For this review, take the finished solid that the model builds, in its own axes (mm). Face numbers are marked on the shaded views. A direction names the side the tool comes from. Coordinates: 2 decimals unless noted, no trailing zeros. Write each loop counter-clockwise with the first axis right and the second up, starting at its lowest first coordinate (ties: lowest second). Pieces come first, ordered by that corner, then holes.
1) Mouldability with a two-part tool opening along Z and no side actions: class the marked faces 5, 6 and 7 as pulls with the +Z half, pulls with the -Z half, needs draft (parallel to the pull), parting line crosses it, or undercut.
2) Insertion check: P1, Ø3, axis at y = 15, z = 25, coming from the -X side (3 decimals); P2, Ø3, axis at x = 24.5, z = 20.5, coming from the -Y side; P3, Ø12, axis at x = 38.5, z = 27, coming from the +Y side; P4, Ø8, axis at y = 41.5, z = 32.5, coming from the -X side. Each pin has a flat end and moves straight along its axis. Give the tip position at first contact, or say it passes through.
3) We need section C-C on y = 21.5. Write out the cut boundary in (x, z) (3 decimals), then the cut area to 3 significant figures.
4) We need section D-D on x = 102.5. Write out the cut boundary in (y, z) (3 decimals).
5) For the marked faces 1, 2, 3 and 4, list the 3-axis set-ups (+Z, -Z, +X, -X, +Y, -Y) from which the entire face can be reached by the end or side of a thin tool; tool diameter is ignored.
6) We need section B-B on x = 43. Write out the cut boundary in (y, z) (3 decimals).
7) To check wall thickness, follow line 1 along Z through (x, y) = (6, 47) (3 decimals); line 2 along X through (y, z) = (-34, 3.5) (3 decimals); line 3 along Y through (x, z) = (11.5, 22). State the ranges of each line that lie inside material, in increasing order.
8) We need section A-A on y = -47.5. Write out the cut boundary in (x, z) (3 decimals).
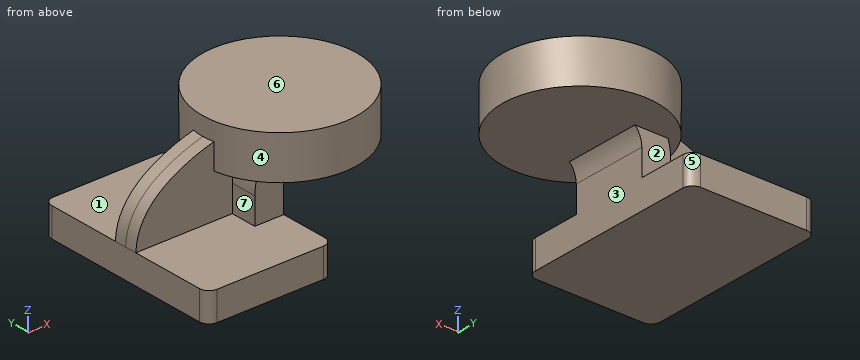
from build123d import *

# Parameters (mm, degrees)
F1_DEPTH = 63.5
F2_DEPTH = 25.4
F3_DEPTH = 7.9375
F5_R     = 6.35


with BuildPart() as f1:
    # F0 (on Front) → F1 (new body, symmetric)
    with BuildSketch(Plane.XZ):
        Polygon((22.225, 9.525), (-41.275, 9.525), (-41.275, -9.525), (41.275, -9.525), (41.275, 9.525), align=None)
    extrude(amount=F1_DEPTH, both=True)

    # F0 (on Front) → F2 (join, symmetric)
    with BuildSketch(Plane.XZ):
        with BuildLine():
            Line((22.225, 27.0002), (22.225, 9.525))
            Line((22.225, 9.525), (41.275, 9.525))
            Line((41.275, 9.525), (41.275, 27.0002))
            ThreePointArc((41.275, 27.0002), (45.92468, 38.22552), (57.15, 42.8752))
            Line((57.15, 42.8752), (60.325, 42.8752))
            Line((60.325, 42.8752), (60.325, 61.9252))
            Line((60.325, 61.9252), (57.15, 61.9252))
            add(Edge.make_bspline(
                [(52.862794, 61.661064), (54.29404, 61.759798), (55.723602, 61.847744), (57.15, 61.9252)],
                knots=[108.118875, 108.118875, 108.118875, 108.118875, 111.504536, 111.504536, 111.504536, 111.504536], degree=3))
            ThreePointArc((52.862794, 61.661064), (30.982403, 50.130537), (22.225, 27.0002))
        make_face()
    extrude(amount=F2_DEPTH, both=True)

    # F0 (on Front) → F3 (join, symmetric)
    with BuildSketch(Plane.XZ):
        with BuildLine():
            add(Edge.make_bspline(
                [(-41.275, 9.525), (-40.267717, 44.353871), (7.156863, 58.508061), (52.862794, 61.661064)],
                knots=[0, 0, 0, 0, 108.118875, 108.118875, 108.118875, 108.118875], degree=3))
            Line((-41.275, 9.525), (22.225, 9.525))
            Line((22.225, 9.525), (22.225, 27.0002))
            ThreePointArc((22.225, 27.0002), (30.982403, 50.130537), (52.862794, 61.661064))
        make_face()
    extrude(amount=F3_DEPTH, both=True)

    # F0 (on Front) → F4 (revolve)
    with BuildSketch(Plane.XZ):
        Polygon((60.325, 66.675), (60.325, 61.9252), (60.325, 42.8752), (60.325, 38.1), (111.125, 38.1), (111.125, 66.675), align=None)
    revolve(axis=Axis((60.325, 0, 52.3875), (0, 0, -1)))

    # F5
    f5_edges = [f1.edges().sort_by_distance(p)[0] for p in [
        (-41.275, -63.5, 0),
        (41.275, -63.5, 0),
        (41.275, 63.5, 0),
        (-41.275, 63.5, 0),
    ]]
    fillet(f5_edges, radius=F5_R)


solid = f1.part
Result:
1. face 5: needs draft
1. face 6: pulls with the +Z half
1. face 7: undercut
2. P1: stops at x = 22.225
2. P2: stops at y = -25.4
2. P3: stops at y = 25.4
2. P4: passes through
3. outline: (-41.275, -9.525) - (41.275, -9.525) - (41.275, 27) arc R15.875 cw to (45.801, 38.1) - (106.351, 38.1) - (106.351, 66.675) - (14.299, 66.675) - (14.299, 38.1) - (24.036, 38.1) arc R34.925 ccw to (22.225, 27) - (22.225, 9.525) - (-41.275, 9.525) - close
3. area: 4,760 mm2
4. outline: (-28.318, 38.1) - (28.318, 38.1) - (28.318, 66.675) - (-28.318, 66.675) - close
5. face 1: -X, +Y
5. face 2: +X, -X, +Y
5. face 3: -Z, +X, +Y, -Y
5. face 4: +Z
6. outline: (-47.754, 38.1) - (-25.4, 38.1) - (-25.4, 34.197) - (25.4, 34.197) - (25.4, 38.1) - (47.754, 38.1) - (47.754, 66.675) - (-47.754, 66.675) - close
7. line 1: z = -9.525 to 9.525
7. line 2: x = -41.275 to 41.275
7. line 3: y = -7.94 to 7.94
8. outline: (-41.275, -9.525) - (41.275, -9.525) - (41.275, 9.525) - (-41.275, 9.525) - close; (42.314, 38.1) - (78.336, 38.1) - (78.336, 66.675) - (42.314, 66.675) - close
